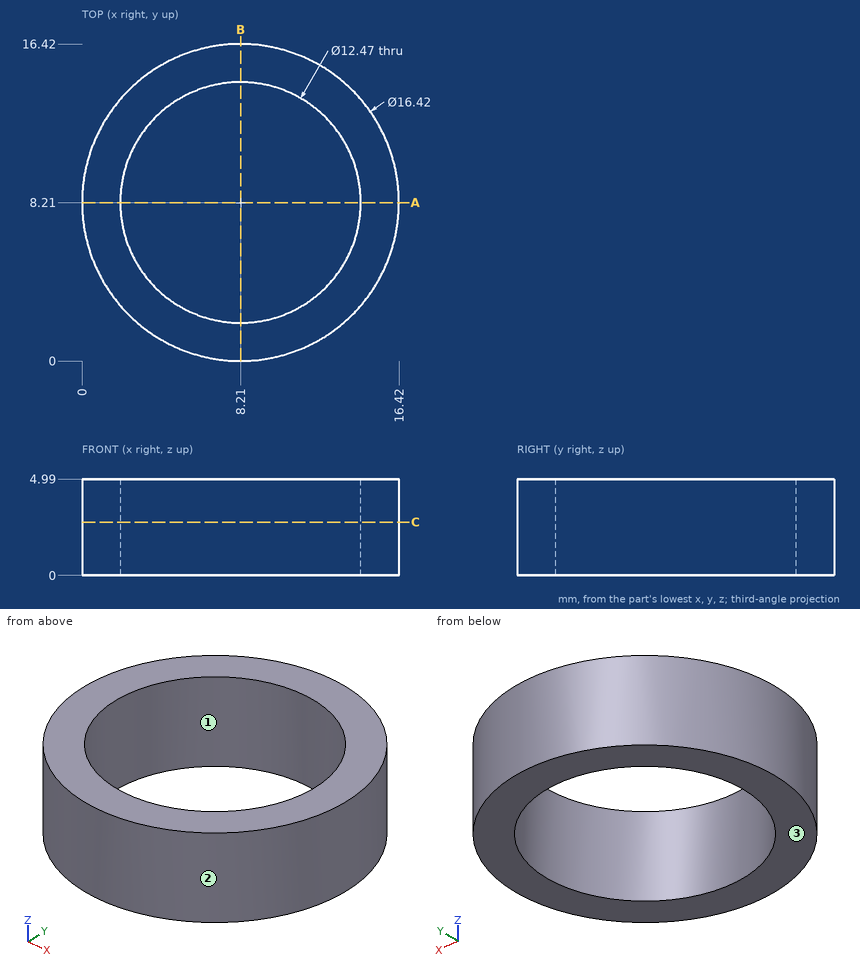
The figure shows three views and two pictorial views of one solid part (mm, origin at its lowest corner). Answer the questions. Round coordinates to 2 decimals unless told otherwise and drop trailing zeros. Write each loop counter-clockwise with the first axis right and the second up, starting at its lowest first coordinate (ties: lowest second). Pieces come first, ordered by that corner, then holes. Notation, with made-up numbers: M 67,9.5 L 90,9.5 A29 cw 90,39.5 Z; hole C -10,-10.75 d3. An arc over 180 degrees is marked long. Write each question's results on one line, items separated by ' | '. Start each with the question number.
(1) Find the intervals of material crossed by line 1 (Y direction, x = 8.21, z = 3.65) (3 decimals); line 2 (X direction, y = 10.25, z = 3.65); line 3 (X direction, y = 8.5, z = 2.8), in increasing order.
(2) The part is cut by section A-A, the plane y = 8.21. Write down the section's boundary in (x, z) (3 decimals), and give its area (3 significant figures).
(3) The part is cut by section C-C, the plane z = 2.75. Write down the section's boundary in (x, y) (3 decimals), and give its area (3 significant figures).
(4) Each of these flat-tipped pins is pushed along its axis until it touches: P1, Ø2, axis at x = 13.5, z = 1, coming from the +Y side; P2, Ø1.5, axis at y = 2.5, z = 2, coming from the -X side. Where does it stop, or does it pass through?
(5) Determine the mould class of the marked faces 1, 2 and 3 for opening direction X: +X half, -X half, draft (parallel to the pull), parting line (faces both ways), or undercut.
Worked answers:
1) line 1: y = 0 to 1.975, 14.445 to 16.42 | line 2: x = 0.26 to 2.32, 14.1 to 16.16 | line 3: x = 0.01 to 1.98, 14.44 to 16.41
2) outline: M 0,0 L 1.975,0 L 1.975,4.99 L 0,4.99 Z; M 14.445,0 L 16.42,0 L 16.42,4.99 L 14.445,4.99 Z | area: 19.7 mm²
3) outline: C 8.21,8.21 d16.42; hole C 8.21,8.21 d12.47 | area: 89.6 mm²
4) P1: stops at y = 15.21 | P2: stops at x = 1.67
5) face 1: undercut | face 2: parting line | face 3: draft
